Geometry: see drawing. Coordinates: mm, zero at the bounding-box minimum. A direction names the side the tool comes from. Give positions to 0.01 mm unless a question says otherwise; leave off trailing zeros. Order: outer loops, then holes, each group sorted by start corner. A loop starts at its lowest first (then second) coordinate and runs counter-clockwise, first axis right, second up. Notation, with made-up numbers: M 54,-26.5 L 66,-26.5 A13 cw 66,-16.5 Z; hole C -33.75,20 d5. An arc over 180 degrees is marked long. Answer as a JSON object with one key per item and string values. Group by question number.
1. Section query C-C (x = 16). Output: boundary loops of the cut face in (y, z) (3 decimals).
2. Material intervals for L1, parallel to X at y = 13.5, z = 37.5; L2, parallel to X at y = 41, z = 73.5, sorted ascending. Write a range as [from, to].
3. Pin query (flat end, axial travel): P1, Ø24, axis at x = 36.5, y = 14, coming from the -Z side. Return the tip coordinate at first contact, or that it passes through.
4. Section query B-B (z = 37). Output: boundary loops of the cut face in (x, y) (3 decimals), plus the area to 3 significant figures.
5. Pull-direction query (Z, two-part tool) for the marked faces 3, 4, 5 and 6; classes: +Z half, -Z half, draft (parallel to the pull), parting line (faces both ways), or undercut.
6. Set-up query: the marked faces 1 and 2. Return all of +Z, -Z, +X, -X, +Y, -Y with unobstructed straight access to the full face (end or side cutting, diameter ignored); none if empty.
7. Section query A-A (y = 37.5). Output: boundary loops of the cut face in (x, z), plus the area to 3 significant figures.
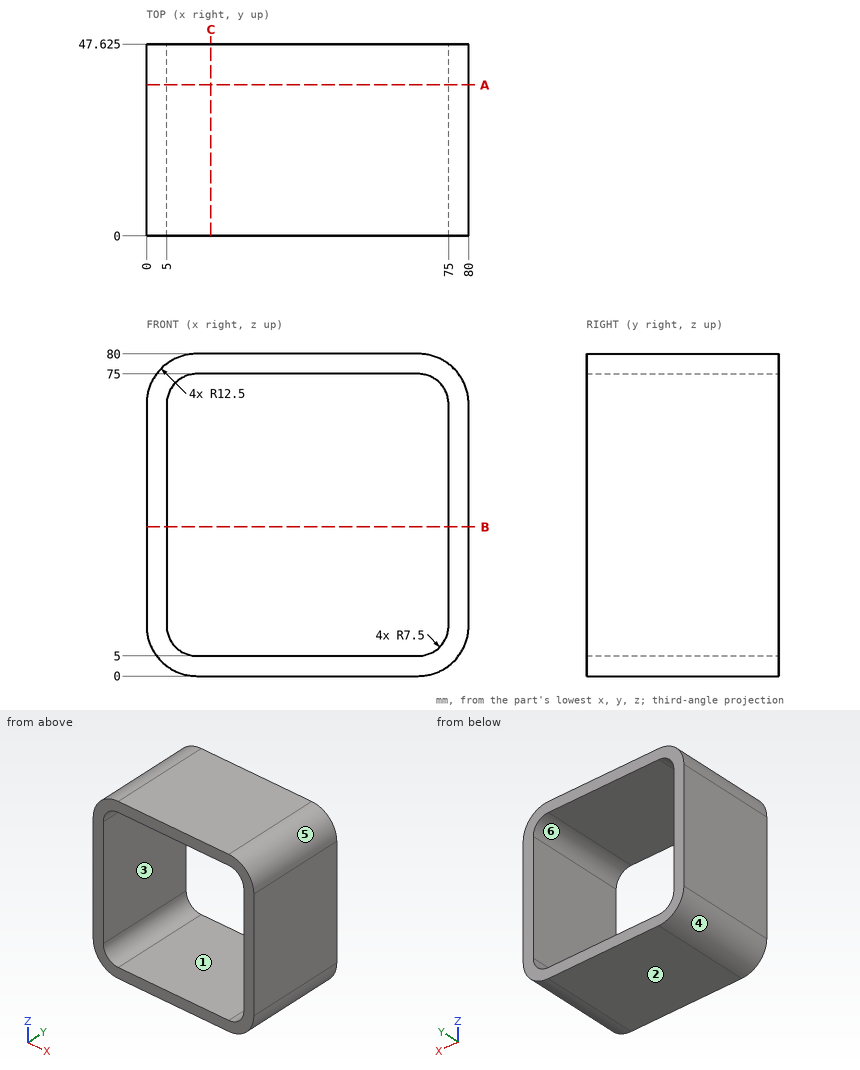
Answer sheet:
{
 "1": {"outline": "M 0,0 L 47.625,0 L 47.625,5 L 0,5 Z; M 0,75 L 47.625,75 L 47.625,80 L 0,80 Z"},
 "2": {"L1": "[0, 5], [75, 80]", "L2": "[1.53, 8], [72, 78.47]"},
 "3": {"P1": "z = 0"},
 "4": {"outline": "M 0,0 L 5,0 L 5,47.625 L 0,47.625 Z; M 75,0 L 80,0 L 80,47.625 L 75,47.625 Z", "area": "476 mm^2"},
 "5": {"face 3": "undercut", "face 4": "-Z half", "face 5": "+Z half", "face 6": "undercut"},
 "6": {"face 1": "+Y, -Y", "face 2": "-Z, +X, -X, +Y, -Y"},
 "7": {"outline": "M 0,12.5 A12.5 ccw 12.5,0 L 67.5,0 A12.5 ccw 80,12.5 L 80,67.5 A12.5 ccw 67.5,80 L 12.5,80 A12.5 ccw 0,67.5 Z; hole M 5,12.5 A7.5 ccw 12.5,5 L 67.5,5 A7.5 ccw 75,12.5 L 75,67.5 A7.5 ccw 67.5,75 L 12.5,75 A7.5 ccw 5,67.5 Z", "area": "1,410 mm^2"}
}
